Check sheet for the modelled part. Datum: model origin and axes. Units: mm. A direction names the side the tool comes from. Coordinates: 2 decimals unless noted, no trailing zeros. Loops run counter-clockwise (first coordinate to the right, second up) from the corner with the lowest first, then second, coordinate; pieces in that order, holes last. Notation, with made-up numbers: (-6, -33) -> (17, -33) arc R24 cw to (17, 6) -> close; hole circle Ø7 at (66, 85). An arc over 180 degrees is marked (long way). Use CSV: the item, a comma, the result in double quotes. Start each with the question number.
1. Gauge pin test, flat ends, axial feed: pin 1 (1.5 mm diameter, centred on x = 1, z = 1, fed in from -Y); pin 2 (1 mm diameter, centred on x = 2.5, y = 0.5, fed in from -Z); pin 3 (1.5 mm diameter, centred on x = 3, z = 1, fed in from -Y). Record the tip position at first contact, or that the pin passes through.
2. Release check for a two-part mould opening along Z. For faces 3 (the face through (0.73, -0.41, 0.19)), 4 (the face through (6.33, 0.08, -0.26)), 5 (the face through (1.6, -1, 1)) record: pulls with the +Z half, pulls with the -Z half, needs draft (parallel to the pull), parting line crosses it, or undercut.
3. Sectioned sample at A-A, the plane x = 3.75. Record the cut outline in (y, z).
4. Sectioned sample at B-B, the plane x = 6. Record the cut outline in (y, z).
5. Set-up check for faces 1 (the face through (0.73, -0.19, -0.41)), 2 (the face through (4, 0, -1)): record each of +Z, -Z, +X, -X, +Y, -Y from which the full face is reachable in a straight line by a thin tool's end or side.
6. Thickness scan on L1, parallel to Z at x = 0.75, y = -0.3; L2, parallel to Y at x = 3, z = 0.35; L3, parallel to Z at x = 5.75, y = 0.45. Record the ranges inside material, lowest first.
```python
from build123d import *

# Parameters (mm, degrees)
FILLET2_R = 0.2


with BuildPart() as part:
    # Sketch1 → Revolve1 (revolve)
    with BuildSketch(Plane(origin=(0, 0, 0), x_dir=(1, 0, 0), z_dir=(0, 1, 0))):
        with BuildLine():
            Line((1.6, 1), (6.6, 1))
            Line((6.6, 1), (6.6, 0))
            Line((6.6, 0), (0, 0))
            ThreePointArc((0, 0), (0.12318754, 0.742622052), (0.479554358, 1.405694727))
            ThreePointArc((0.479554358, 1.405694727), (0.97590539, 1.809326647), (1.6, 1.95))
            Line((1.6, 1.95), (1.6, 1))
        make_face()
    revolve(axis=Axis((-13.629268293, 0, 0), (1, 0, 0)))

    # Fillet2
    fillet2_edges = [part.edges().sort_by_distance(p)[0] for p in [
        (1.6, 0, 1),
    ]]
    fillet(fillet2_edges, radius=FILLET2_R)

    # Sketch4 → Cut-Revolve1 (revolve, cut)
    with BuildSketch(Plane(origin=(0, 0, 0), x_dir=(1, 0, 0), z_dir=(0, 1, 0))):
        Polygon((7.333454633, 0), (7.333454633, 21), (-14.4, 21), (6.6, 0), align=None)
    revolve(axis=Axis((4.782773752, 0, 0), (1, 0, 0)), mode=Mode.SUBTRACT)

    # Sketch2 → Cut-Loft1 section 0
    with BuildSketch(Plane(origin=(0, 0, 0), x_dir=(0, 0, -1), z_dir=(1, 0, 0)), mode=Mode.PRIVATE) as cut_loft1_s0:
        Polygon((-0.3125, 0.3125), (-1.25, 0.3125), (-1.25, -0.3125), (-0.3125, -0.3125), (-0.3125, -1.25), (0.3125, -1.25), (0.3125, -0.3125), (1.25, -0.3125), (1.25, 0.3125), (0.3125, 0.3125), (0.3125, 1.25), (-0.3125, 1.25), align=None)
    loft([Vertex(1.85, 0, 0), cut_loft1_s0.sketch], mode=Mode.SUBTRACT)


solid = part.part
```
Completed:
1,pin 1,"y = -1.9"
1,pin 2,"z = -1"
1,pin 3,"y = -0.97"
2,face 3,"undercut"
2,face 4,"parting line crosses it"
2,face 5,"needs draft"
3,outline,"circle Ø2 at (0, 0)"
4,outline,"circle Ø1.2 at (0, 0)"
5,face 1,"-X"
5,face 2,"+X"
6,L1,"-1.64 to -0.19, 0.19 to 1.64"
6,L2,"-0.94 to 0.94"
6,L3,"-0.72 to 0.72"
